Check sheet for the modelled part. Datum: model origin and axes. Units: mm. Give positions to 0.01 mm unless a question says otherwise; leave off trailing zeros. Loops run counter-clockwise (first coordinate to the right, second up) from the corner with the lowest first, then second, coordinate; pieces in that order, holes last. Notation, with made-up numbers: (41.25, 65.5) - (61.25, 65.5) arc R33 ccw to (61.25, 95.5) - close; hole circle Ø7 at (70.25, 9). An arc over 180 degrees is marked (long way). Answer in a Markdown table with one row per item. Add a question column.
(1) Thickness scan on L1, parallel to X at y = -317.5, z = 0.5; L2, parallel to Y at x = 2, z = -7.25; L3, parallel to Z at x = -0.25, y = -378.5. Record the ranges inside material, lowest first.
(2) Sectioned sample at B-B on x = 0. Enter the section's corners in (y, z), then the cut area to 3 significant figures.
(3) Sectioned sample at A-A on z = 0. Enter the section's corners in (x, y), then the cut area to 3 significant figures.
(4) Go/stop test with flat-tipped pins: P1, Ø6.5, axis at y = -465.5, z = 0, coming from the -X side; P2, Ø2, axis at x = -6, y = -361, coming from the -Z side; P3, Ø10, axis at y = -417.5, z = -7.5, coming from the -X side; P4, Ø6, axis at x = 3.5, z = 0, coming from the -Y side. Record where each tip stops, or that it passes through.
(5) Sectioned sample at C-C on y = -361. Enter the section's corners in (x, z).
from build123d import *

# Parameters (mm, degrees)
F0_R     = 10
F1_DEPTH = 424
F2_SIZE  = 1
F3_W     = 6
F3_H     = 6
F4_DEPTH = 100


with BuildPart() as f1:
    # F0 (on Front) → F1 (new body)
    with BuildSketch(Plane.XZ):
        Circle(F0_R)
    extrude(amount=F1_DEPTH)

    # F2
    f2_edges = [f1.edges().sort_by_distance(p)[0] for p in [
        (-10, 0, 0),
        (-10, -424, 0),
    ]]
    chamfer(f2_edges, length=F2_SIZE)

    # F3 (on face) → F4 (join)
    with BuildSketch(Plane.XZ.offset(424)):
        Rectangle(F3_W, F3_H)
    extrude(amount=F4_DEPTH)


solid = f1.part
Reply:
| question | item | result |
|---|---|---|
| 1 | L1 | -9.99 to 9.99 |
| 1 | L2 | -424 to 0 |
| 1 | L3 | -10 to 10 |
| 2 | outline | (-524, -3) - (-424, -3) - (-424, -9) - (-423, -10) - (-1, -10) - (0, -9) - (0, 9) - (-1, 10) - (-423, 10) - (-424, 9) - (-424, 3) - (-524, 3) - close |
| 2 | area | 9,080 mm^2 |
| 3 | outline | (-10, -423) - (-9, -424) - (-3, -424) - (-3, -524) - (3, -524) - (3, -424) - (9, -424) - (10, -423) - (10, -1) - (9, 0) - (-9, 0) - (-10, -1) - close |
| 3 | area | 9,080 mm^2 |
| 4 | P1 | x = -3 |
| 4 | P2 | z = -8.66 |
| 4 | P3 | x = -9.68 |
| 4 | P4 | y = -524 |
| 5 | outline | circle Ø20 at (0, 0) |
